from build123d import *

# Parameters (mm, degrees)
SKIZZE1_W                       = 2.5
SKIZZE1_H                       = 3
SKIZZE1_W_2                     = 7
SKIZZE1_H_2                     = 7
SKIZZE1_R                       = 1.25
SKIZZE1_H_3                     = 22.5
SKIZZE1_R_2                     = 1.5
AUFSATZ_LINEAR_AUSTRAGEN1_DEPTH = 3
SKIZZE2_W                       = 2
SKIZZE2_H                       = 29.5
SKIZZE2_W_2                     = 1.5
SKIZZE2_H_2                     = 3
AUFSATZ_LINEAR_AUSTRAGEN2_DEPTH = 3
SKIZZE3_W                       = 1
SKIZZE3_H                       = 1
SKIZZE3_H_2                     = 2
SKIZZE3_W_2                     = 13
SKIZZE3_H_3                     = 29.5
SCHNITT_LINEAR_AUSTRAGEN1_DEPTH = 10
SKIZZE4_W                       = 0.8
SKIZZE4_H                       = 1.999250504
SKIZZE4_H_2                     = 2
AUFSATZ_LINEAR_AUSTRAGEN3_DEPTH = 3
SKIZZE5_R                       = 1.6
SCHNITT_LINEAR_AUSTRAGEN2_DEPTH = 3


with BuildPart() as part:
    # Skizze1 → Aufsatz-Linear austragen1 (new body)
    # profile 1 of 5: a face of its own
    with BuildSketch(Plane.XY):
        with Locations((4.75, 14.75)):
            Rectangle(SKIZZE1_W, SKIZZE1_H)
    # profile 2 of 5: a face of its own
    with BuildSketch(Plane.XY):
        with Locations((0, 14.75)):
            Rectangle(SKIZZE1_W_2, SKIZZE1_H)
    # profile 3 of 5: a face of its own
    with BuildSketch(Plane.XY):
        with Locations((-4.75, 14.75)):
            Rectangle(SKIZZE1_W, SKIZZE1_H)
    # profile 4 of 5: a face of its own
    with BuildSketch(Plane.XY):
        with Locations((0, 9.75)):
            Rectangle(SKIZZE1_W_2, SKIZZE1_H_2)
        with Locations((0, 11.25)):
            Circle(SKIZZE1_R, mode=Mode.SUBTRACT)
    # profile 5 of 5: a face of its own
    with BuildSketch(Plane.XY):
        with Locations((0, -5)):
            Rectangle(SKIZZE1_W_2, SKIZZE1_H_3)
        with Locations((0, -13.95)):
            Circle(SKIZZE1_R_2, mode=Mode.SUBTRACT)
        with Locations((0, 3.55)):
            Circle(SKIZZE1_R_2, mode=Mode.SUBTRACT)
    extrude(amount=AUFSATZ_LINEAR_AUSTRAGEN1_DEPTH)

    # Skizze2 → Aufsatz-Linear austragen2 (add)
    with BuildSketch(Plane(origin=(0, 0, 0), x_dir=(-1, 0, 0), z_dir=(0, 0, -1))):
        with Locations((-4.5, -1.5)):
            Rectangle(SKIZZE2_W, SKIZZE2_H)
        with Locations((4.5, -1.5)):
            Rectangle(SKIZZE2_W, SKIZZE2_H)
        with Locations((6.75, 14.75)):
            Rectangle(SKIZZE2_W_2, SKIZZE2_H_2)
        with Locations((-6.75, 14.75)):
            Rectangle(SKIZZE2_W_2, SKIZZE2_H_2)
    extrude(amount=-AUFSATZ_LINEAR_AUSTRAGEN2_DEPTH)

    # Skizze3 → Schnitt-Linear austragen1 (cut)
    with BuildSketch(Plane.XY.offset(3)):
        with Locations((-7, 15.75)):
            Rectangle(SKIZZE3_W, SKIZZE3_H)
        with Locations((-7, 14.25)):
            Rectangle(SKIZZE3_W, SKIZZE3_H_2)
        with Locations((0, 15.75)):
            Rectangle(SKIZZE3_W_2, SKIZZE3_H)
        with Locations((7, 15.75)):
            Rectangle(SKIZZE3_W, SKIZZE3_H)
        with Locations((7, 14.25)):
            Rectangle(SKIZZE3_W, SKIZZE3_H_2)
        with Locations((5, -1.5)):
            Rectangle(SKIZZE3_W, SKIZZE3_H_3)
        with Locations((-5, -1.5)):
            Rectangle(SKIZZE3_W, SKIZZE3_H_3)
    extrude(amount=-SCHNITT_LINEAR_AUSTRAGEN1_DEPTH, mode=Mode.SUBTRACT)

    # Skizze4 → Aufsatz-Linear austragen3 (add)
    with BuildSketch(Plane.XY.offset(3)):
        Polygon((-7.3, 15.25), (-7.3, 16.05), (7.3, 16.05), (7.3, 15.25), (6.5, 15.25), (-6.5, 15.25), align=None)
        with Locations((-6.9, 14.250374748)):
            Rectangle(SKIZZE4_W, SKIZZE4_H)
        Polygon((-4.5, 13.25), (-5.3, 13.25), (-5.3, -16.271198208), (-4.5, -16.271198208), (-4.5, -16.25), align=None)
        Polygon((5.3, -16.271198208), (5.3, 13.25), (4.5, 13.25), (4.5, -16.25), (4.5, -16.271198208), align=None)
        with Locations((6.9, 14.25)):
            Rectangle(SKIZZE4_W, SKIZZE4_H_2)
    extrude(amount=-AUFSATZ_LINEAR_AUSTRAGEN3_DEPTH)

    # Skizze5 → Schnitt-Linear austragen2 (cut)
    with BuildSketch(Plane.XY.offset(3)):
        with Locations((0, 11.25)):
            Circle(SKIZZE5_R)
        with Locations((0, 3.55)):
            Circle(SKIZZE5_R)
        with Locations((0, -13.95)):
            Circle(SKIZZE5_R)
    extrude(amount=-SCHNITT_LINEAR_AUSTRAGEN2_DEPTH, mode=Mode.SUBTRACT)


solid = part.part
For this review, take the finished solid that the model builds, in its own axes (mm). A direction names the side the tool comes from. Coordinates: 2 decimals unless noted, no trailing zeros. Order: outer loops, then holes, each group sorted by start corner. A loop starts at its lowest first (then second) coordinate and runs counter-clockwise, first axis right, second up. Notation, with made-up numbers: (47.25, -31.5) - (91.25, -31.5) arc R18 ccw to (91.25, 1.5) - close; hole circle Ø7 at (71, 89.5). An arc over 180 degrees is marked (long way). Use one line per item in the form item = value.
Q1. Consider section B-B (z = 1.75). Give the number of separate pieces and of enclosed holes in the cut face, then the cut area to 3 significant figures.
Checked values:
separate_pieces = 1
enclosed_holes = 3
area = 329 mm2
Q2. Draft analysis for pull direction X (two halves, no side actions). For faces 1 (the cylindrical face through (-0.35, 1.99, 1.52)), 2 (the flat face through (-7.3, 15, 2)), 3 (the flat face through (5.3, -2, 2)), state which applies: +X half, -X half, draft (parallel to the pull), parting line (faces both ways), or undercut.
Checked values:
face_1 = undercut
face_2 = -X half
face_3 = +X half
Q3. Consider section D-D (y = 4). Give the boundary of the cut face in (x, z), then the cut area to 3 significant figures.
Checked values:
outline = (-5.3, 0) - (-1.54, 0) - (-1.54, 3) - (-5.3, 3) - close; (1.54, 0) - (5.3, 0) - (5.3, 3) - (1.54, 3) - close
area = 22.6 mm2
Q4. For probe 1 along Y at (x, z) = (0, 0.8); probe 2 along X at (y, z) = (-4.5, 1.75); probe 3 along Y at (x, z) = (-5.5, 1.1), list the stretches that pass through material, from the lowest coordinate up. Write a range as from..to.
Checked values:
probe_1 = -16.25..-15.55, -12.35..1.95, 5.15..9.65, 12.85..16.05
probe_2 = -5.3..5.3
probe_3 = 13.25..16.05
Q5. Consider section C-C (x = 0). Give the boundary of the cut face in (y, z), then the cut area to 3 significant figures.
Checked values:
outline = (-16.25, 0) - (-15.55, 0) - (-15.55, 3) - (-16.25, 3) - close; (-12.35, 0) - (1.95, 0) - (1.95, 3) - (-12.35, 3) - close; (5.15, 0) - (9.65, 0) - (9.65, 3) - (5.15, 3) - close; (12.85, 0) - (16.05, 0) - (16.05, 3) - (12.85, 3) - close
area = 68.1 mm2
Q6. Consider section A-A (y = -13.95). Give the boundary of the cut face in (x, z).
Checked values:
outline = (-5.3, 0) - (-1.6, 0) - (-1.6, 3) - (-5.3, 3) - close; (1.6, 0) - (5.3, 0) - (5.3, 3) - (1.6, 3) - close
Q7. For P1, Ø0.6, axis at x = -6, z = 1.5, coming from the -Y side; P2, Ø1.5, axis at x = 0, z = 1, coming from the -Y side; P3, Ø0.6, axis at x = -7, z = 1.5, coming from the -Y side, all flat-tipped, find the tip position at first contact; note any pin that passes through.
Checked values:
P1 = 13.25
P2 = -16.25
P3 = 13.25
Q8. For faces 4 (the flat face through (-5.3, -1, 2)), 5 (the cylindrical face through (-0.208, 12.836, 1.521)), 6 (the flat face through (6, 13.25, 2)), list the 3-axis set-ups (+Z, -Z, +X, -X, +Y, -Y) from which the entire face can be reached by the end or side of a thin tool; tool diameter is ignored.
Checked values:
face_4 = +Z, -Z, -X, -Y
face_5 = +Z, -Z
face_6 = +Z, -Z, +X, -Y
